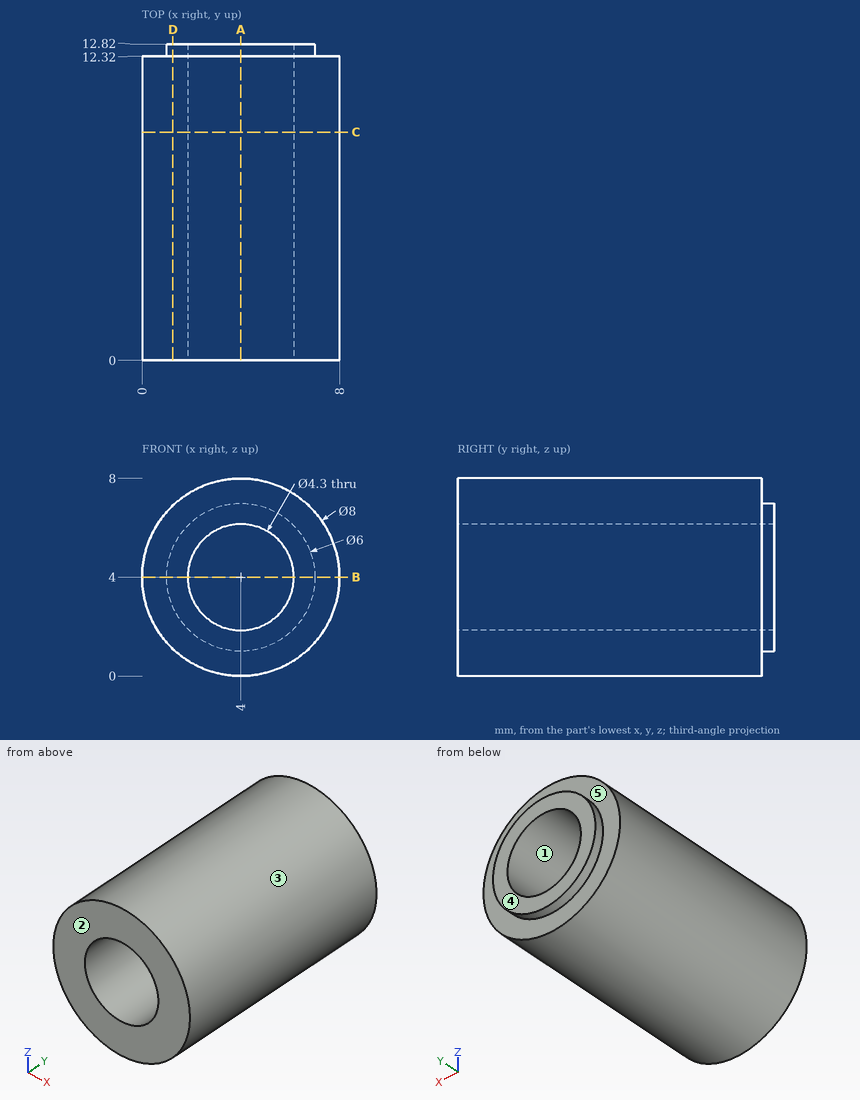
Geometry check sheet. Reference: drawing and pictorial views, mm from the part's lowest x, y, z. A direction names the side the tool comes from. Give positions to 0.01 mm unless a question says otherwise; leave off trailing zeros. Write each loop counter-clockwise with the first axis right and the second up, starting at its lowest first coordinate (ties: lowest second). Pieces come first, ordered by that corner, then holes.
Item 1: Cross-section at C-C (y = 9.25). Enter the section's corners in (x, z), and give its area (3 significant figures).
Item 2: Draft check along Z on the marked faces 1, 2 and 3. Enter one of: released by +Z, released by -Z, zero draft, split by the parting line, or undercut.
Item 3: Access from +Z, -Z, +X, -X, +Y, -Y to the whole of each face (thin tool, end or side, straight path). Record for the marked faces 4 and 5.
Item 4: Cross-section at A-A (x = 4). Enter the section's corners in (y, z), and give its area (3 significant figures).
Item 5: Gauge pin test, flat ends, axial feed: pin 1 (3 mm diameter, centred on y = 5.5, z = 6, fed in from +X); pin 2 (3.5 mm diameter, centred on x = 4, z = 4, fed in from -Y). Record the tip position at first contact, or that the pin passes through.
Item 6: Cross-section at D-D (x = 1.25). Enter the section's corners in (y, z).
Item 7: Cross-section at B-B (z = 4). Enter the section's corners in (x, y).
Item 8: Scan lines: L1, parallel to Z at x = 4, y = 5; L2, parallel to Y at x = 5.5, z = 7.25; L3, parallel to Z at x = 3.25, y = 5.25. Record each from-to range of solid material in increasing order.
Report:
1. outline: circle Ø8 at (4, 4); hole circle Ø4.3 at (4, 4)
1. area: 35.7 mm2
2. face 1: undercut
2. face 2: zero draft
2. face 3: split by the parting line
3. face 4: +Z, -Z, +X, -X, +Y
3. face 5: +Y
4. outline: (0, 0) - (12.32, 0) - (12.32, 1) - (12.82, 1) - (12.82, 1.85) - (0, 1.85) - close; (0, 6.15) - (12.82, 6.15) - (12.82, 7) - (12.32, 7) - (12.32, 8) - (0, 8) - close
4. area: 46.4 mm2
5. pin 1: stops at x = 7.97
5. pin 2: passes through
6. outline: (0, 1.1) - (12.32, 1.1) - (12.32, 2.8) - (12.82, 2.8) - (12.82, 5.2) - (12.32, 5.2) - (12.32, 6.9) - (0, 6.9) - close
7. outline: (0, 0) - (1.85, 0) - (1.85, 12.82) - (1, 12.82) - (1, 12.32) - (0, 12.32) - close; (6.15, 0) - (8, 0) - (8, 12.32) - (7, 12.32) - (7, 12.82) - (6.15, 12.82) - close
8. L1: z = 0 to 1.85, 6.15 to 8
8. L2: y = 0 to 12.32
8. L3: z = 0.07 to 1.99, 6.01 to 7.93
